Geometry: final body of the model. Coordinates: model frame, mm. Face numbers are marked on the shaded views. A direction names the side the tool comes from. Round coordinates to 2 decimals unless told otherwise and drop trailing zeros. Order: outer loops, then holes, each group sorted by start corner. A loop starts at its lowest first (then second) coordinate and runs counter-clockwise, first axis right, second up. Notation, with made-up numbers: (-23, 41.25) -> (-5, 41.25) arc R22 cw to (-5, 51.25) -> close; hole circle Ø1 at (44.5, 63.5). An arc over 180 degrees is marked (long way). Put each result on its own line as item: value.
```python
from build123d import *

# Parameters (mm, degrees)
SKETCH1_W               = 150
SKETCH1_H               = 60
SKETCH1_W_2             = 141
SKETCH1_H_2             = 52
BOSS_EXTRUDE1_DEPTH     = 20
SKETCH2_W               = 150
SKETCH2_H               = 60
BOSS_EXTRUDE2_DEPTH     = 4
SKETCH3_W               = 132
SKETCH3_H               = 17
CUT_EXTRUDE1_DEPTH      = 16
SKETCH4_R               = 1.75
CUT_EXTRUDE3_DEPTH      = 21
CUT_EXTRUDE3_DEPTH_BACK = 5
CUT_EXTRUDE4_START      = -20
SKETCH5_R               = 3
CUT_EXTRUDE4_DEPTH      = 20


with BuildPart() as part:
    # Sketch1 → Boss-Extrude1 (new body)
    with BuildSketch(Plane.XY):
        with Locations((75, 30)):
            Rectangle(SKETCH1_W, SKETCH1_H)
        with Locations((75, 30)):
            Rectangle(SKETCH1_W_2, SKETCH1_H_2, mode=Mode.SUBTRACT)
    extrude(amount=BOSS_EXTRUDE1_DEPTH)

    # Sketch2 → Boss-Extrude2 (add)
    with BuildSketch(Plane.XY.offset(20)):
        with Locations((75, 30)):
            Rectangle(SKETCH2_W, SKETCH2_H)
    extrude(amount=BOSS_EXTRUDE2_DEPTH)

    # Sketch3 → Cut-Extrude1 (cut)
    with BuildSketch(Plane.XZ):
        with Locations((75, 8.5)):
            Rectangle(SKETCH3_W, SKETCH3_H)
    extrude(amount=-CUT_EXTRUDE1_DEPTH, mode=Mode.SUBTRACT)

    # Sketch4 → Cut-Extrude3 (cut, two sides)
    with BuildSketch(Plane(origin=(0, 0, 20), x_dir=(-1, 0, 0), z_dir=(0, 0, -1))) as cut_extrude3_sk:
        with Locations((-140.25, 54.625)):
            Circle(SKETCH4_R)
        with Locations((-9.75, 54.625)):
            Circle(SKETCH4_R)
        with Locations((-9.75, 5.375)):
            Circle(SKETCH4_R)
        with Locations((-140.25, 5.375)):
            Circle(SKETCH4_R)
    extrude(amount=CUT_EXTRUDE3_DEPTH, mode=Mode.SUBTRACT)
    extrude(cut_extrude3_sk.sketch, amount=-CUT_EXTRUDE3_DEPTH_BACK, mode=Mode.SUBTRACT)

    # Sketch5 → Cut-Extrude4 (cut)
    with BuildSketch(Plane(origin=(0, 0, 0), x_dir=(-1, 0, 0), z_dir=(0, 0, -1)).offset(CUT_EXTRUDE4_START)):
        with Locations((-140.25, 5.375)):
            Circle(SKETCH5_R)
        with Locations((-9.75, 5.375)):
            Circle(SKETCH5_R)
        with Locations((-140.25, 54.625)):
            Circle(SKETCH5_R)
        with Locations((-9.75, 54.625)):
            Circle(SKETCH5_R)
    extrude(amount=CUT_EXTRUDE4_DEPTH, mode=Mode.SUBTRACT)


solid = part.part
```
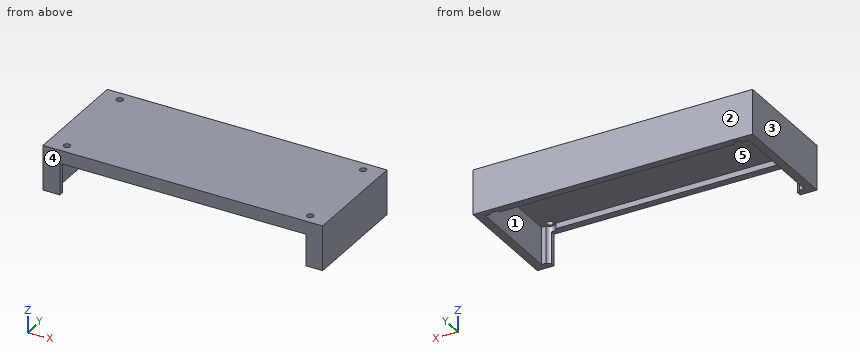
1. Draft query along Y for the marked faces 1, 2 and 3. Return one class per face: +Y half, -Y half, draft (parallel to the pull), parting line (faces both ways), or undercut.
Ans:
face 1: undercut
face 2: +Y half
face 3: draft
2. Cut plane A-A on x = 117. Return loops of the section in (y, z), and give its area (3 significant figures).
Ans:
outline: (0, 17) -> (4, 17) -> (4, 20) -> (56, 20) -> (56, 0) -> (60, 0) -> (60, 24) -> (0, 24) -> close
area: 332 mm²
3. Contact query for flat-ended pins moving along their axis: P1, Ø3, axis at x = 83, y = 34.5, coming from the -Z side; P2, Ø6, axis at x = 73, z = 8, coming from the -Y side; P3, Ø2, axis at x = 58, y = 3, coming from the -Z side. Output: stop coordinate, or through.
Ans:
P1: z = 20
P2: y = 56
P3: z = 17
4. Set-up query: the marked faces 4 and 5. Return all of +Z, -Z, +X, -X, +Y, -Y with unobstructed straight access to the full face (end or side cutting, diameter ignored); none if empty.
Ans:
face 4: +Z, -Z, +X, -X, -Y
face 5: -Z
5. Material intervals for probe 1 along Y at (x, z) = (140.25, 20.8) (3 decimals); probe 2 along X at (y, z) = (37.5, 16.5); probe 3 along X at (y, z) = (56, 21), sorted ascending.
Ans:
probe 1: 0 to 3.625, 7.125 to 52.875, 56.375 to 60
probe 2: 0 to 4.5, 145.5 to 150
probe 3: 0 to 8.67, 10.83 to 139.17, 141.33 to 150
6. Cut plane C-C on z = 13. Return loops of the section in (x, y) (3 decimals), and give its area (3 significant figures).
Ans:
outline: (0, 0) -> (9, 0) -> (9, 2.47) arc R3 cw to (7.084, 4) -> (4.5, 4) -> (4.5, 56) -> (7.084, 56) arc R3 cw to (12.416, 56) -> (137.584, 56) arc R3 cw to (142.916, 56) -> (145.5, 56) -> (145.5, 4) -> (142.916, 4) arc R3 cw to (141, 2.47) -> (141, 0) -> (150, 0) -> (150, 60) -> (0, 60) -> close
area: 1,120 mm²
7. Cut plane B-B on y = 42. Return loops of the section in (x, z), and give its area (3 significant figures).
Ans:
outline: (0, 0) -> (4.5, 0) -> (4.5, 20) -> (145.5, 20) -> (145.5, 0) -> (150, 0) -> (150, 24) -> (0, 24) -> close
area: 780 mm²
